Autodesk Inventor part; units mm, degrees
ref_plane "YZ Plane" through (0, 0, 0) normal (1, 0, 0) x (0, 1, 0)
ref_plane "XZ Plane" through (0, 0, 0) normal (0, 1, 0) x (-1, 0, 0)
ref_plane "XY Plane" through (0, 0, 0) normal (0, 0, 1) x (1, 0, 0)
sketch "Sketch1" plane through (0, 0, 0) normal (0, 1, 0) x (-1, 0, 0)
  line L0 (0, 0) -> (0, -5.2929)
  line L1 (0, -5.2929) -> (-0.7071, -6)
  line L2 (-0.7071, -6) -> (-2, -6)
  line L3 (-2, -6) -> (-2, -5.5)
  line L4 (-2, -5.5) -> (-2.7, -5.5)
  line L5 (-2.7, -5.5) -> (-2.7, -6)
  line L6 (-2.7, -6) -> (-34.2, -6)
  line L7 (-34.2, -6) -> (-34.2, 0)
  line L8 (-34.2, 0) -> (0, 0)
  line L9 (-68.4, 0) -> (-68.4, -5.2929)
  line L10 (-68.4, -5.2929) -> (-67.6929, -6)
  line L11 (-67.6929, -6) -> (-66.4, -6)
  line L12 (-66.4, -6) -> (-66.4, -5.5)
  line L13 (-66.4, -5.5) -> (-65.7, -5.5)
  line L14 (-65.7, -5.5) -> (-65.7, -6)
  line L15 (-65.7, -6) -> (-34.2, -6)
  line L16 (-68.4, 0) -> (-34.2, 0)
  dimension "d0" = 6
  dimension "d1" = 0.7
  dimension "d2" = 2
  dimension "d3" = 0.5
  dimension "d4" = 135
  dimension "d5" = 1
  dimension "d8" = 31.5
revolve "Revolution1" add sketch "Sketch1" angle 360 about axis through (68.4, 0, 0) along (-1, 0, 0)
properties part number "Shatf_piston"
Geometry: final body of the model. Coordinates: model frame, mm. A direction names the side the tool comes from. Coordinates: 2 decimals unless noted, no trailing zeros. Order: outer loops, then holes, each group sorted by start corner. A loop starts at its lowest first (then second) coordinate and runs counter-clockwise, first axis right, second up.
(1) Section query A-A (x = 42). Return the cut outline in (y, z).
(2) First-contact query: pin 1 (1 mm diameter, centred on x = 28.5, y = 2.5, fed in from -Z); pin 2 (1 mm diameter, centred on x = 42.5, z = -4.5, fed in from +Y). Flat tips, straight axial feed; report the tip coordinate or a pass-through.
(3) Access query for faces 5 (the face through (65.7, 5, -3)), 6 (the face through (1, 0, 6)). Directions: +Z, -Z, +X, -X, +Y, -Y. A direction counts if a zero-diameter tool reaches every point of the face in a straight line with its end or side. Return the directions, or none.
(4) Material intervals for probe 1 along X at (y, z) = (3.5, 4.5); probe 2 along Z at (x, y) = (43, -0.25), sorted ascending.
(5) Draft query along X for faces 1 (the face through (0, 0, 0)), 2 (the face through (66.4, 5, -3)), 3 (the face through (2.7, 5, -3)), 4 (the face through (35, 0, 6)). Return one class per face: pulls with the +X half, pulls with the -X half, needs draft (parallel to the pull), parting line crosses it, or undercut.
Solution:
1. outline: circle Ø12 at (0, 0)
2. pin 1: stops at z = -5.66
2. pin 2: stops at y = 4.47
3. face 5: none
3. face 6: +X, -X
4. probe 1: x = 0.41 to 2, 2.7 to 65.7, 66.4 to 67.99
4. probe 2: z = -5.99 to 5.99
5. face 1: pulls with the -X half
5. face 2: undercut
5. face 3: undercut
5. face 4: needs draft
